Input: part model. Units: mm. Frame: model coordinates. A direction names the side the tool comes from. Coordinates: 2 decimals unless noted, no trailing zeros. Order: outer loops, then holes, each group sorted by start corner. A loop starts at its lowest first (then second) coordinate and runs counter-clockwise, first axis right, second up.
from build123d import *

# Parameters (mm, degrees)
SKETCH2_W               = 40.64
SKETCH2_H               = 127
BOSS_EXTRUDE1_DEPTH     = 6.35
M6_CLEARANCE_HOLE1_D    = 6.6
SKETCH5_W               = 7.0505
SKETCH5_H               = 127
CUT_EXTRUDE1_DEPTH      = 1
CUT_EXTRUDE1_DEPTH_BACK = 7.35
SKETCH6_W               = 27.8745
SKETCH6_H               = 3.175
CUT_EXTRUDE2_DEPTH      = 7.35
SKETCH7_W               = 6.35
SKETCH7_H               = 4.7625
CUT_EXTRUDE3_DEPTH      = 7.35


with BuildPart() as part:
    # Sketch2 → Boss-Extrude1 (new body)
    with BuildSketch(Plane.XY):
        with Locations((20.32, 63.5)):
            Rectangle(SKETCH2_W, SKETCH2_H)
    extrude(amount=BOSS_EXTRUDE1_DEPTH)

    # M6 Clearance Hole1 (through all)
    with Locations(Plane.XY.offset(6.35)):
        with Locations((17.4625, 31.75), (17.4625, 95.25)):
            Hole(M6_CLEARANCE_HOLE1_D / 2)

    # Sketch5 → Cut-Extrude1 (cut, two sides)
    with BuildSketch(Plane.XY.offset(6.35)) as cut_extrude1_sk:
        with Locations((3.52525, 63.5)):
            Rectangle(SKETCH5_W, SKETCH5_H)
    extrude(amount=CUT_EXTRUDE1_DEPTH, mode=Mode.SUBTRACT)
    extrude(cut_extrude1_sk.sketch, amount=-CUT_EXTRUDE1_DEPTH_BACK, mode=Mode.SUBTRACT)

    # Sketch6 → Cut-Extrude2 (cut, through all)
    with BuildSketch(Plane.XY.offset(6.35)):
        Polygon((7.0505, 123.825), (7.0505, 120.65), (37.30625, 120.65), (37.30625, 127), (34.925, 127), (34.925, 123.825), align=None)
        with Locations((20.98775, 125.4125)):
            Rectangle(SKETCH6_W, SKETCH6_H)
        Polygon((37.30625, 66.675), (7.0505, 66.675), (7.0505, 63.5), (34.925, 63.5), (34.925, 60.325), (7.0505, 60.325), (7.0505, 57.15), (37.30625, 57.15), align=None)
        with Locations((20.98775, 61.9125)):
            Rectangle(SKETCH6_W, SKETCH6_H)
        Polygon((37.30625, 0), (37.30625, 6.35), (7.0505, 6.35), (7.0505, 3.175), (34.925, 3.175), (34.925, 0), align=None)
        with Locations((20.98775, 1.5875)):
            Rectangle(SKETCH6_W, SKETCH6_H)
    extrude(amount=-CUT_EXTRUDE2_DEPTH, mode=Mode.SUBTRACT)

    # Sketch7 → Cut-Extrude3 (cut, through all)
    with BuildSketch(Plane.XY.offset(6.35)):
        with Locations((31.115, 8.73125)):
            Rectangle(SKETCH7_W, SKETCH7_H)
        Polygon((27.94, 11.1125), (34.29, 11.1125), (34.29, 6.35), (34.671, 6.35), (34.671, 11.4935), (27.559, 11.4935), (27.559, 6.35), (27.94, 6.35), align=None)
        Polygon((34.671, 6.35), (34.29, 6.35), (27.94, 6.35), (27.559, 6.35), (27.559, 5.969), (34.671, 5.969), align=None)
        with Locations((31.115, 54.76875)):
            Rectangle(SKETCH7_W, SKETCH7_H)
        Polygon((34.671, 57.15), (34.29, 57.15), (34.29, 52.3875), (27.94, 52.3875), (27.94, 57.15), (27.559, 57.15), (27.559, 52.0065), (34.671, 52.0065), align=None)
        Polygon((27.94, 57.15), (34.29, 57.15), (34.671, 57.15), (34.671, 57.531), (27.559, 57.531), (27.559, 57.15), align=None)
        Polygon((34.671, 66.675), (34.29, 66.675), (27.94, 66.675), (27.559, 66.675), (27.559, 66.294), (34.671, 66.294), align=None)
        with Locations((31.115, 69.05625)):
            Rectangle(SKETCH7_W, SKETCH7_H)
        Polygon((27.94, 71.4375), (34.29, 71.4375), (34.29, 66.675), (34.671, 66.675), (34.671, 71.8185), (27.559, 71.8185), (27.559, 66.675), (27.94, 66.675), align=None)
        with Locations((31.115, 118.26875)):
            Rectangle(SKETCH7_W, SKETCH7_H)
        Polygon((27.559, 115.5065), (34.671, 115.5065), (34.671, 120.65), (34.29, 120.65), (34.29, 115.8875), (27.94, 115.8875), (27.94, 120.65), (27.559, 120.65), align=None)
        Polygon((34.29, 120.65), (34.671, 120.65), (34.671, 121.031), (27.559, 121.031), (27.559, 120.65), (27.94, 120.65), align=None)
    extrude(amount=-CUT_EXTRUDE3_DEPTH, mode=Mode.SUBTRACT)


solid = part.part
Item 1: Ray query, probe 1 along Y at (x, z) = (24, 1) (3 decimals); probe 2 along Y at (x, z) = (16, 4) (3 decimals); probe 3 along Y at (x, z) = (18, 4.25) (3 decimals). Return the intervals inside material, ascending.
Response values:
probe 1: y = 6.35 to 57.15, 66.675 to 120.65
probe 2: y = 6.35 to 28.792, 34.708 to 57.15, 66.675 to 92.292, 98.208 to 120.65
probe 3: y = 6.35 to 28.494, 35.006 to 57.15, 66.675 to 91.994, 98.506 to 120.65
Item 2: Draft query along X for faces 1 (the face through (39, 127, 3)), 2 (the face through (14.414, 30.486, 3.131)), 3 (the face through (7.05, 31, 3)). Return one class per face: pulls with the +X half, pulls with the -X half, needs draft (parallel to the pull), parting line crosses it, or undercut.
Response values:
face 1: needs draft
face 2: undercut
face 3: pulls with the -X half
Item 3: Cut plane A-A on y = 117. Return loops of the section in (x, z), then the cut area to 3 significant figures.
Response values:
outline: (7.05, 0) - (27.56, 0) - (27.56, 6.35) - (7.05, 6.35) - close; (34.67, 0) - (40.64, 0) - (40.64, 6.35) - (34.67, 6.35) - close
area: 168 mm2
Item 4: Pin query (flat end, axial travel): pin 1 Ø1.5 at (x, z) = (33, 4) entering from +Y; pin 2 Ø1.3 at (x, z) = (35.5, 4) entering from +Y; pin 3 Ø2 at (x, z) = (28, 1) entering from -Y. Return the tip coordinate at first contact, or that it passes through.
Response values:
pin 1: stops at y = 115.51
pin 2: stops at y = 120.65
pin 3: stops at y = 6.35
Item 5: Cut plane C-C on z = 3. Count the separate pieces of the cut face and the enclosed holes in it, then the cut area to 3 significant figures.
Response values:
separate pieces: 1
enclosed holes: 2
area: 3,380 mm2
Item 6: Access query for faces 4 (the face through (36, 57.15, 3)), 5 (the face through (34.671, 69, 3)), 6 (the face through (17, 120.65, 3)), 7 (the face through (31, 115.506, 3)). Directions: +Z, -Z, +X, -X, +Y, -Y. A direction counts if a zero-diameter tool reaches every point of the face in a straight line with its end or side. Return the directions, or none.
Response values:
face 4: +Z, -Z, -X
face 5: +Z, -Z
face 6: +Z, -Z, -X, +Y
face 7: +Z, -Z, +Y
Item 7: Cut plane D-D on x = 18. Return loops of the section in (y, z) (3 decimals).
Response values:
outline: (6.35, 0) - (28.494, 0) - (28.494, 6.35) - (6.35, 6.35) - close; (35.006, 0) - (57.15, 0) - (57.15, 6.35) - (35.006, 6.35) - close; (66.675, 0) - (91.994, 0) - (91.994, 6.35) - (66.675, 6.35) - close; (98.506, 0) - (120.65, 0) - (120.65, 6.35) - (98.506, 6.35) - close
Item 8: Cut plane B-B on x = 25. Return loops of the section in (y, z) (3 decimals).
Response values:
outline: (6.35, 0) - (57.15, 0) - (57.15, 6.35) - (6.35, 6.35) - close; (66.675, 0) - (120.65, 0) - (120.65, 6.35) - (66.675, 6.35) - close
